```python
from build123d import *

# Parameters (mm, degrees)
F1_DEPTH = 63.5
F0_W     = 25.4
F0_H     = 19.05
F2_DEPTH = 25.4
F3_DEPTH = 7.9375
F5_R     = 6.35


with BuildPart() as f1:
    # F0 (on Front) → F1 (new body, symmetric)
    with BuildSketch(Plane.XZ):
        Polygon((41.275, -9.525), (41.275, 9.525), (22.225, 9.525), (-41.275, 9.525), (-41.275, -9.525), align=None)
    extrude(amount=F1_DEPTH, both=True)

    # F0 (on Front) → F2 (join, symmetric)
    with BuildSketch(Plane.XZ):
        with Locations((73.025, 52.4002)):
            Rectangle(F0_W, F0_H)
        with BuildLine():
            Line((22.225, 9.525), (41.275, 9.525))
            Line((41.275, 9.525), (41.275, 27.0002))
            ThreePointArc((41.275, 27.0002), (45.9246798487, 38.2255201513), (57.15, 42.8752))
            Line((57.15, 42.8752), (60.325, 42.8752))
            Line((60.325, 42.8752), (60.325, 61.9252))
            Line((60.325, 61.9252), (57.15, 61.9252))
            ThreePointArc((57.15, 61.9252), (32.4542956671, 51.6959043329), (22.225, 27.0002))
            Line((22.225, 27.0002), (22.225, 9.525))
        make_face()
    extrude(amount=F2_DEPTH, both=True)

    # F0 (on Front) → F3 (join, symmetric)
    with BuildSketch(Plane.XZ):
        with BuildLine():
            Line((-41.275, 9.525), (22.225, 9.525))
            Line((22.225, 9.525), (22.225, 27.0002))
            ThreePointArc((22.225, 27.0002), (32.4542956671, 51.6959043329), (57.15, 61.9252))
            add(Edge.make_bspline(
                [(-41.275, 9.525), (-42.6979027689, 25.6473943591), (11.1759584397, 66.0527870059), (57.15, 61.9252)],
                knots=[0, 0, 0, 0, 111.5045361635, 111.5045361635, 111.5045361635, 111.5045361635], degree=3))
        make_face()
    extrude(amount=F3_DEPTH, both=True)

    # F0 (on Front) → F4 (revolve)
    with BuildSketch(Plane.XZ):
        Polygon((85.725, 61.9252), (85.725, 42.8752), (85.725, 38.1), (111.125, 38.1), (111.125, 66.675), (85.725, 66.675), align=None)
    revolve(axis=Axis((85.725, 0, 52.3875), (0, 0, 1)))

    # F5
    f5_edges = [f1.edges().sort_by_distance(p)[0] for p in [
        (41.275, -63.5, 0),
        (-41.275, -63.5, 0),
        (41.275, 63.5, 0),
        (-41.275, 63.5, 0),
    ]]
    fillet(f5_edges, radius=F5_R)


solid = f1.part
```
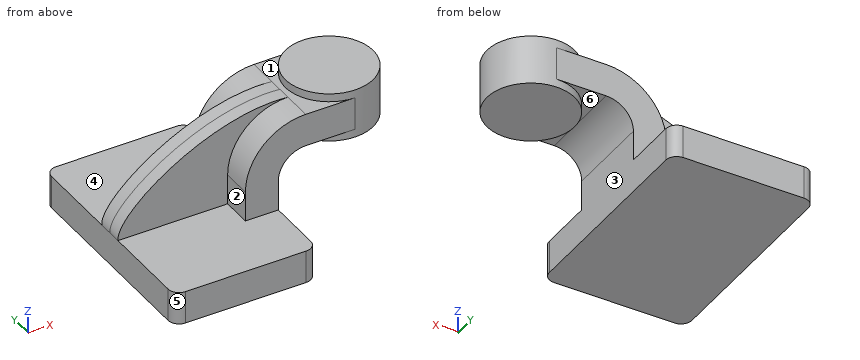
Input: part model. Units: mm. Frame: model coordinates. Face numbers are marked on the shaded views. A direction names the side the tool comes from. Give positions to 0.01 mm unless a question says otherwise; leave off trailing zeros. Write each loop counter-clockwise with the first axis right and the second up, starting at its lowest first coordinate (ties: lowest second). Pieces come first, ordered by that corner, then holes. Notation, with made-up numbers: (-18, 42.5) - (25, 42.5) arc R27 ccw to (25, 77.5) - close; hole circle Ø10 at (74, -24.5). An arc over 180 degrees is marked (long way). Write item = value, one per line. Start each with the question number.
1. First-contact query: pin 1 Ø16.5 at (x, y) = (-7.5, -44.5) entering from +Z (3 decimals); pin 2 Ø8 at (x, y) = (35, 28) entering from +Z; pin 3 Ø19 at (y, z) = (13.5, 16) entering from -X; pin 4 Ø6 at (x, z) = (-13, 33.5) entering from -Y. Flat tips, straight axial feed; report the tip coordinate or a pass-through.
2. Ray query, L1, parallel to Z at x = 58, y = 7.5; L2, parallel to X at y = -42, z = 0 (3 decimals); L3, parallel to Z at x = 73, y = -4 (3 decimals). Return the intervals inside material, ascending.
3. Mould query, pull axis X, two halves, no side actions, for the marked faces 4, 5 and 6. Classes: released by +X, released by -X, zero draft, split by the parting line, or undercut.
4. Section query C-C, the plane y = -32. Output: boundary loops of the cut face in (x, z) (3 decimals), then the cut area to 3 significant figures.
5. Section query A-A, the plane y = 18. Output: boundary loops of the cut face in (x, z) (3 decimals), then the cut area to 3 significant figures.
6. Section query B-B, the plane x = 97.5. Output: boundary loops of the cut face in (y, z) (3 decimals), then the cut area to 3 significant figures.
7. Access query for the marked faces 1, 2 and 3. Directions: +Z, -Z, +X, -X, +Y, -Y. A direction counts if a zero-diameter tool reaches every point of the face in a straight line with its end or side. Return the directions, or none.
Check sheet entries:
q1.pin_1 = 9.525
q1.pin_2 = 56.23
q1.pin_3 = -41.3
q1.pin_4 = -7.94
q2.L1 = 42.88 to 61.93
q2.L2 = -41.275 to 41.275
q2.L3 = 38.1 to 66.675
q3.face_4 = zero draft
q3.face_5 = released by -X
q3.face_6 = undercut
q4.outline = (-41.275, -9.525) - (41.275, -9.525) - (41.275, 9.525) - (-41.275, 9.525) - close
q4.area = 1,570 mm2
q5.outline = (-41.275, -9.525) - (41.275, -9.525) - (41.275, 27) arc R15.875 cw to (57.15, 42.875) - (67.804, 42.875) - (67.804, 38.1) - (103.646, 38.1) - (103.646, 66.675) - (67.804, 66.675) - (67.804, 61.925) - (57.15, 61.925) arc R34.925 ccw to (22.225, 27) - (22.225, 9.525) - (-41.275, 9.525) - close
q5.area = 3,890 mm2
q6.outline = (-22.506, 38.1) - (22.506, 38.1) - (22.506, 66.675) - (-22.506, 66.675) - close
q6.area = 1,290 mm2
q7.face_1 = +Z
q7.face_2 = +Z, -X, -Y
q7.face_3 = -Z, +X, +Y, -Y
